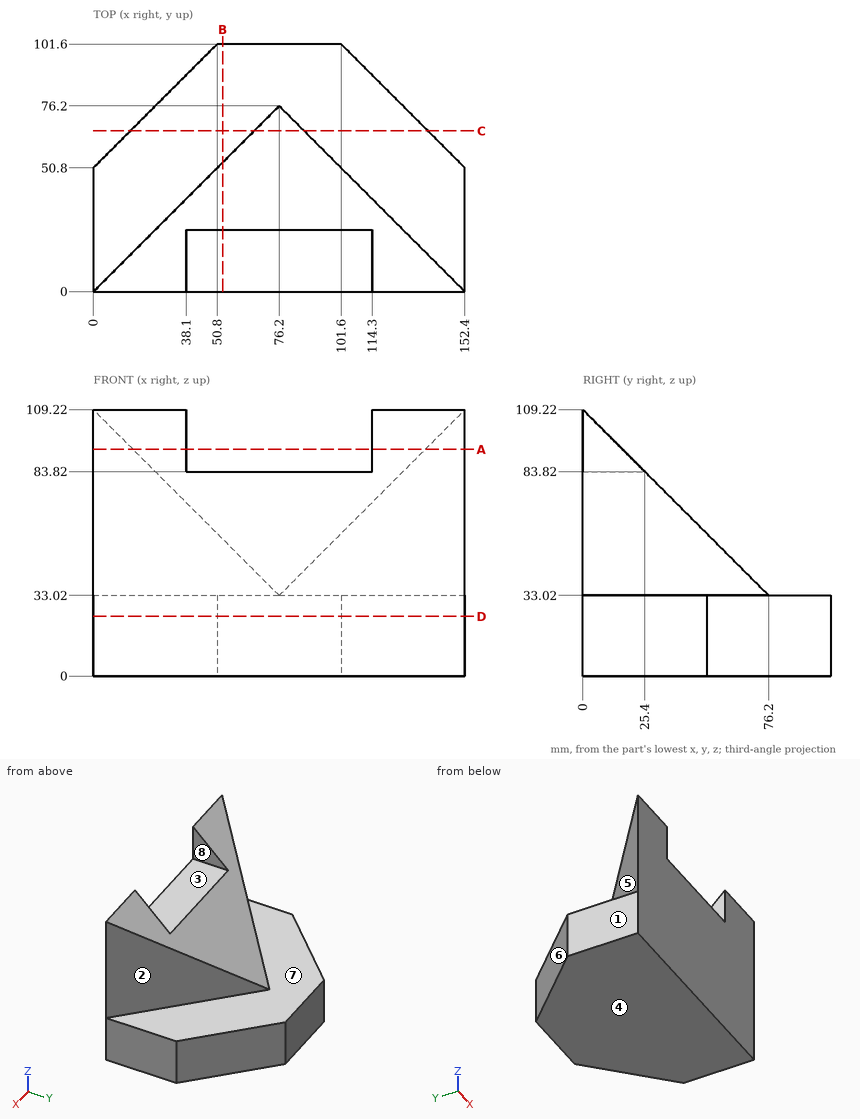
Answer from the drawing. Dimensions are ordinates in mm from the lowest x, y and z of the part. A direction names the side the tool comes from. Round coordinates to 2 decimals unless told otherwise and drop trailing zeros. Write each loop counter-clockwise with the first axis right and the second up, starting at its lowest first coordinate (ties: lowest second). Pieces come first, ordered by that corner, then holes. Notation, with made-up numbers: M 78,45 L 92,45 A19 ccw 92,78 Z; hole C 83,-4 d2. An arc over 180 degrees is marked long. One line per item, written item: value.
Q1. Find section A-A on z = 93. Write down the section's boundary in (x, y), plus the area to 3 significant figures.
Data:
outline: M 0,0 L 38.1,0 L 38.1,16.22 L 16.22,16.22 Z; M 114.3,0 L 152.4,0 L 136.18,16.22 L 114.3,16.22 Z
area: 973 mm2
Q2. Find section B-B on x = 53. Write down the section's boundary in (y, z), plus the area to 3 significant figures.
Data:
outline: M 0,0 L 101.6,0 L 101.6,33.02 L 53,33.02 L 53,56.22 L 25.4,83.82 L 0,83.82 Z
area: 5,670 mm2
Q3. For a pull along X with two mould halves and no side action, classify the marked faces 1, 2 and 3 as +X half, -X half, draft (parallel to the pull), parting line (faces both ways), or undercut.
Data:
face 1: -X half
face 2: +X half
face 3: undercut
Q4. Flat-ended cylindrical pins translate along their axes: pin 1 Ø3 at (x, y) = (102.5, 73) entering from +Z; pin 2 Ø2 at (x, y) = (35.5, 30) entering from +Z; pin 3 Ø2 at (y, z) = (26.5, 72) entering from -X. Find the tip coordinate at first contact, or state that the pin passes through.
Data:
pin 1: z = 33.02
pin 2: z = 80.22
pin 3: x = 25.5
Q5. Which of the six approach directions +Z, -Z, +X, -X, +Y, -Y give full straight-line access (tool end or side, diameter ignored) to the marked faces 4, 5, 6, 7 and 8?
Data:
face 4: -Z, +X, -X, +Y, -Y
face 5: +Z, -X, +Y
face 6: +Z, -Z, -X, +Y
face 7: +Z, +Y
face 8: +Z, +Y, -Y
Q6. Straight lines are drawn through the part: line 1 (Z direction, x = 115, y = 62.5); line 2 (Y direction, x = 127, z = 20); line 3 (X direction, y = 11.5, z = 84.5). For each, find the intervals that lie inside material, in ascending order. Write a range as [from, to].
Data:
line 1: [0, 33.02]
line 2: [0, 76.2]
line 3: [11.5, 38.1], [114.3, 140.9]
Q7. Find section C-C on y = 66. Write down the section's boundary in (x, z).
Data:
outline: M 15.2,0 L 137.2,0 L 137.2,33.02 L 86.4,33.02 L 86.4,43.22 L 66,43.22 L 66,33.02 L 15.2,33.02 Z
Q8. Find section D-D on z = 24.5. Write down the section's boundary in (x, y), plus the area to 3 significant figures.
Data:
outline: M 0,0 L 152.4,0 L 152.4,50.8 L 101.6,101.6 L 50.8,101.6 L 0,50.8 Z
area: 12,900 mm2
